Source: CAD feature listing. Evaluate the final solid. Frame: model axes, mm. Face numbers are marked on the shaded views. A direction names the side the tool comes from. Give positions to 0.01 mm unless a question says otherwise; leave off trailing zeros. Order: outer loops, then holes, each group sorted by start corner. A loop starts at its lowest first (then second) coordinate and runs counter-clockwise, first axis right, second up. Notation, with made-up numbers: (72.5, 63) - (111.5, 63) arc R26 cw to (111.5, 92) - close; hole circle Ø10 at (44.25, 82). An arc over 180 degrees is marked (long way). Use CSV: the item, a comma, the result in double quotes.
```python
from build123d import *

# Parameters (mm, degrees)
SKETCH1_W           = 10
SKETCH1_H           = 9
SKETCH1_R           = 0.603114575
BOSS_EXTRUDE1_DEPTH = 1
SKETCH2_W           = 1.840309862
SKETCH2_H           = 6.861155246
BOSS_EXTRUDE2_DEPTH = 1.25


with BuildPart() as part:
    # Sketch1 → Boss-Extrude1 (new body)
    with BuildSketch(Plane(origin=(0, 0, 0), x_dir=(1, 0, 0), z_dir=(0, 1, 0))):
        Rectangle(SKETCH1_W, SKETCH1_H)
        with Locations(Location((-3.974491731, -1.184022837, 0), (0, 0, 270))):
            Circle(SKETCH1_R, mode=Mode.SUBTRACT)
        with Locations(Location((-3.974491731, 0.493456275, 0), (0, 0, 270))):
            Circle(SKETCH1_R, mode=Mode.SUBTRACT)
        with Locations(Location((-3.974491731, 1.868439153, 0), (0, 0, 270))):
            Circle(SKETCH1_R, mode=Mode.SUBTRACT)
        with Locations(Location((4.08905372, 3.680148348, 0), (0, 0, 270))):
            Circle(SKETCH1_R, mode=Mode.SUBTRACT)
        with Locations(Location((3.855346006, -3.469811406, 0), (0, 0, 270))):
            Circle(SKETCH1_R, mode=Mode.SUBTRACT)
    extrude(amount=BOSS_EXTRUDE1_DEPTH)

    # Sketch2 → Boss-Extrude2 (add)
    with BuildSketch(Plane(origin=(0, 1, 0), x_dir=(1, 0, 0), z_dir=(0, 1, 0))):
        Rectangle(SKETCH2_W, SKETCH2_H)
    extrude(amount=BOSS_EXTRUDE2_DEPTH)


solid = part.part
```
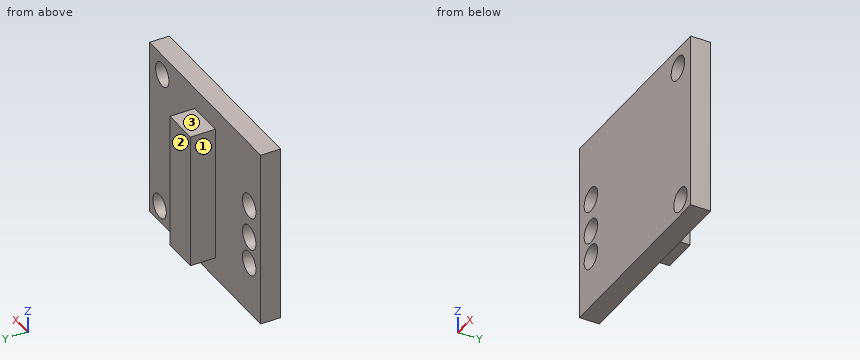
Item 1: Section D-D on y = 0.55. Return the cut outline in (x, z).
Filled in:
outline,"(-5, -4.5) - (5, -4.5) - (5, 4.5) - (-5, 4.5) - close; hole circle Ø1.21 at (-3.97, -1.87); hole circle Ø1.21 at (-3.97, -0.49); hole circle Ø1.21 at (-3.97, 1.18); hole circle Ø1.21 at (3.86, 3.47); hole circle Ø1.21 at (4.09, -3.68)"
Item 2: Set-up query: the marked faces 1, 2 and 3. Return all of +Z, -Z, +X, -X, +Y, -Y with unobstructed straight access to the full face (end or side cutting, diameter ignored); none if empty.
Filled in:
face 1,"+Z, -Z, -X, +Y"
face 2,"+Z, -Z, +X, -X, +Y"
face 3,"+Z, +X, -X, +Y"
Item 3: Section A-A on z = 2. Return the cut outline in (x, y), then the cut area to 3 significant figures.
Filled in:
outline,"(-5, 0) - (5, 0) - (5, 1) - (0.92, 1) - (0.92, 2.25) - (-0.92, 2.25) - (-0.92, 1) - (-5, 1) - close"
area,"12.3 mm2"
Item 4: First-contact query: pin 1 (4.5 mm diameter, centred on x = -1, z = -1, fed in from +Y); pin 2 (0.6 mm diameter, centred on x = 0, y = 1.5, fed in from -Z); pin 3 (1.9 mm diameter, centred on x = -3.97, z = 1.18, fed in from +Y); pin 4 (0.6 mm diameter, centred on y = 1.5, z = -0.5, fed in from +X). Flat tips, straight axial feed; report the tip coordinate or a pass-through.
Filled in:
pin 1,"stops at y = 2.25"
pin 2,"stops at z = -3.43"
pin 3,"stops at y = 1"
pin 4,"stops at x = 0.92"
Item 5: Section B-B on z = -3.75. Return the cut outline in (x, y).
Filled in:
outline,"(-5, 0) - (3.49, 0) - (3.49, 1) - (-5, 1) - close; (4.69, 0) - (5, 0) - (5, 1) - (4.69, 1) - close"
Item 6: Material intervals for line 1 (Z direction, x = -3.75, y = 0.8); line 2 (Y direction, x = 4, z = 1); line 3 (X direction, y = 0.55, z = -2), sorted ascending. Write a range as from..to.
Filled in:
line 1,"z = -4.5..-2.43, -1.31..-1.05, 0.07..0.62, 1.74..4.5"
line 2,"y = 0..1"
line 3,"x = -5..-4.56, -3.39..5"
Item 7: Section C-C on x = 2.5. Return the cut outline in (y, z).
Filled in:
outline,"(0, -4.5) - (1, -4.5) - (1, 4.5) - (0, 4.5) - close"
